For this review, take the finished solid that the model builds, in its own axes (mm). Face numbers are marked on the shaded views. A direction names the side the tool comes from. Give positions to 0.01 mm unless a question says otherwise; leave off trailing zeros. Order: outer loops, then holes, each group sorted by start corner. A loop starts at its lowest first (then second) coordinate and runs counter-clockwise, first axis right, second up. Notation, with made-up numbers: (46, 29.5) - (102, 29.5) arc R30 ccw to (102, 55.5) - close; hole circle Ø4 at (83.25, -8.75). An arc over 180 degrees is marked (long way). One line per item, written item: value.
```python
from build123d import *

# Parameters (mm, degrees)
BOSS_EXTRUDE1_DEPTH = 25.3
CUT_EXTRUDE1_DEPTH  = 25.3
SKETCH14_W          = 4.475703298
SKETCH14_H          = 7.178850836
CUT_EXTRUDE6_DEPTH  = 1.5
SKETCH15_W          = 4.041452
SKETCH15_H          = 7.107257799
CUT_EXTRUDE7_DEPTH  = 1.5
SKETCH16_W          = 5.309940562
SKETCH16_H          = 16
CUT_EXTRUDE8_DEPTH  = 7
SKETCH17_W          = 25.3
SKETCH17_H          = 2.501305671
BOSS_EXTRUDE2_DEPTH = 8.029274
SKETCH18_W          = 25.3
SKETCH18_H          = 2.501305671
BOSS_EXTRUDE3_DEPTH = 8.029274
SKETCH20_W          = 20.1
SKETCH20_H          = 25.3
BOSS_EXTRUDE4_DEPTH = 0.978694
CUT_EXTRUDE9_DEPTH  = 3.48
SKETCH22_W          = 25
SKETCH22_H          = 3.18
CUT_EXTRUDE10_DEPTH = 19.8


with BuildPart() as part:
    # Sketch2 → Boss-Extrude1 (new body)
    with BuildSketch(Plane.XY):
        Polygon((3.031088942, 2.501305671), (4.041452, 2.501305671), (4.041452, 0), (0, 0), (0, 2.501305671), (1.010363, 2.501305671), (2.9e-08, 4.251305671), (1.010363, 6.001305671), (2.9e-08, 7.751305671), (1.010363, 9.501305671), (3.031088942, 9.501305671), (4.041451913, 7.751305671), (3.031088942, 6.001305671), (4.041451913, 4.251305671), align=None)
    extrude(amount=BOSS_EXTRUDE1_DEPTH)

    # Sketch3 → Cut-Extrude1 (cut)
    with BuildSketch(Plane.XY.offset(25.3)):
        Polygon((3.34863159, 7.751305671), (2.684678781, 8.901305671), (1.356773162, 8.901305671), (0.692820352, 7.751305671), (1.356773162, 6.601305671), (2.684678781, 6.601305671), align=None)
        Polygon((3.34863159, 4.251305671), (2.684678781, 5.401305671), (1.356773162, 5.401305671), (0.692820352, 4.251305671), (1.356773162, 3.101305671), (2.684678781, 3.101305671), align=None)
    extrude(amount=-CUT_EXTRUDE1_DEPTH, mode=Mode.SUBTRACT)

    # Sketch14 → Cut-Extrude6 (cut)
    with BuildSketch(Plane(origin=(0, 0, 0), x_dir=(-1, 0, 0), z_dir=(0, 0, -1))):
        with Locations((-1.998569053, 6.096687367)):
            Rectangle(SKETCH14_W, SKETCH14_H)
    extrude(amount=-CUT_EXTRUDE6_DEPTH, mode=Mode.SUBTRACT)

    # Sketch15 → Cut-Extrude7 (cut)
    with BuildSketch(Plane.XY.offset(25.3)):
        with Locations((2.020726, 6.054934571)):
            Rectangle(SKETCH15_W, SKETCH15_H)
    extrude(amount=-CUT_EXTRUDE7_DEPTH, mode=Mode.SUBTRACT)

    # Sketch16 → Cut-Extrude8 (cut)
    with BuildSketch(Plane(origin=(0, 9.501305671, 0), x_dir=(1, 0, 0), z_dir=(0, 1, 0))):
        with Locations((1.902727321, -12.65)):
            Rectangle(SKETCH16_W, SKETCH16_H)
    extrude(amount=-CUT_EXTRUDE8_DEPTH, mode=Mode.SUBTRACT)

    # Sketch17 → Boss-Extrude2 (add)
    with BuildSketch(Plane(origin=(4.041452, 0, 0), x_dir=(0, 0, -1), z_dir=(1, 0, 0))):
        with Locations((-12.65, 1.250652836)):
            Rectangle(SKETCH17_W, SKETCH17_H)
    extrude(amount=BOSS_EXTRUDE2_DEPTH)

    # Sketch18 → Boss-Extrude3 (add)
    with BuildSketch(Plane.ZY):
        with Locations((12.65, 1.250652836)):
            Rectangle(SKETCH18_W, SKETCH18_H)
    extrude(amount=BOSS_EXTRUDE3_DEPTH)

    # Sketch20 → Boss-Extrude4 (add)
    with BuildSketch(Plane.XZ):
        with Locations((2.020726, 12.65)):
            Rectangle(SKETCH20_W, SKETCH20_H)
    extrude(amount=BOSS_EXTRUDE4_DEPTH)

    # Sketch21 → Cut-Extrude9 (cut)
    with BuildSketch(Plane(origin=(0, 2.501305671, 0), x_dir=(1, 0, 0), z_dir=(0, 1, 0))):
        with BuildLine():
            Line((-8.029274, -7.65), (2.010726, -7.65))
            ThreePointArc((2.010726, -7.65), (7.010726, -12.65), (2.010726, -17.65))
            Line((2.010726, -17.65), (-8.029274, -17.65))
            Line((-8.029274, -17.65), (-8.029274, -7.65))
        make_face()
    extrude(amount=-CUT_EXTRUDE9_DEPTH, mode=Mode.SUBTRACT)

    # Sketch22 → Cut-Extrude10 (cut)
    with BuildSketch(Plane.ZY.offset(8.029274)):
        with Locations((12.65, 0.761305671)):
            Rectangle(SKETCH22_W, SKETCH22_H)
    extrude(amount=-CUT_EXTRUDE10_DEPTH, mode=Mode.SUBTRACT)


solid = part.part
```
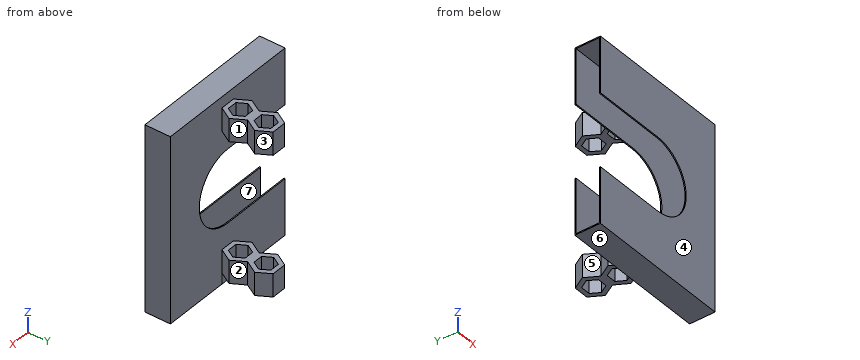
(1) Draft analysis for pull direction Y (two halves, no side actions). For the marked faces 1, 2, 3 and 4, state which applies: pulls with the +Y half, pulls with the -Y half, needs draft (parallel to the pull), parting line crosses it, or undercut.
Answers below:
face 1: undercut
face 2: undercut
face 3: pulls with the +Y half
face 4: pulls with the -Y half
(2) Take a section at D-D (y = 8.25). Write out the cut boundary in (x, z).
Answers below:
outline: (0.29, 1.5) - (0.98, 1.5) - (0.98, 4.65) - (0.29, 4.65) - close; (0.29, 20.65) - (0.98, 20.65) - (0.98, 23.8) - (0.29, 23.8) - close; (3.06, 1.5) - (3.75, 1.5) - (3.75, 4.65) - (3.06, 4.65) - close; (3.06, 20.65) - (3.75, 20.65) - (3.75, 23.8) - (3.06, 23.8) - close
(3) Take a section at A-A (x = -3). Write out the cut boundary in (y, z).
Answers below:
outline: (-0.98, 0) - (2.5, 0) - (2.5, 7.65) - (2.35, 7.65) - (2.35, 0.15) - (-0.83, 0.15) - (-0.83, 7.65) - (-0.98, 7.65) - close; (-0.98, 17.65) - (-0.83, 17.65) - (-0.83, 25.15) - (2.35, 25.15) - (2.35, 17.65) - (2.5, 17.65) - (2.5, 25.3) - (-0.98, 25.3) - close
(4) Wall thickness on line 1 (Z direction, x = 5.5, y = 1.5); line 2 (X direction, y = 1.75, z = 23.75); line 3 (X direction, y = 5, z = 21): over which ranges is each line inside the solid? List them lowest first. Write a range as from..to.
Answers below:
line 1: z = 0..0.15, 25.15..25.3
line 2: x = 11.77..12.07
line 3: x = 0.43..1.13, 2.92..3.61
(5) Take a section at C-C (z = 4). Give the number of separate pieces and of enclosed holes in the cut face, then the cut area to 3 significant figures.
Answers below:
separate pieces: 1
enclosed holes: 2
area: 19.0 mm^2
(6) For P1, Ø2, axis at x = 2, y = 5.5, coming from the -Z side; P2, Ø1, axis at y = 1.5, z = 7.5, coming from the -X side; P3, Ø10, axis at x = 1, z = 18, coming from the +Y side; P4, Ø3, axis at y = 7.5, z = 21, coming from the +X side, all flat-tipped, find the tip position at first contact; note any pin that passes through.
Answers below:
P1: stops at z = 1.5
P2: stops at x = 11.77
P3: stops at y = 9.5
P4: stops at x = 4.04
(7) Machinability: for the marked faces 5, 6 and 7, which of the approach directions +Z, -Z, +X, -X, +Y, -Y give a long, thin tool a straight path to every point of the face, cutting with its end or side? Answer none if there is none.
Answers below:
face 5: +Z, -Z, -X
face 6: -Z, +X, -X, +Y, -Y
face 7: -X
(8) Take a section at B-B (z = 7.25). Write out the cut boundary in (x, y), then the cut area to 3 significant figures.
Answers below:
outline: (-8.03, -0.98) - (12.07, -0.98) - (12.07, 2.5) - (-8.03, 2.5) - (-8.03, 2.35) - (11.77, 2.35) - (11.77, -0.83) - (-8.03, -0.83) - close
area: 6.98 mm^2
